Check sheet for the modelled part. Datum: model origin and axes. Units: mm. Face numbers are marked on the shaded views. A direction names the side the tool comes from. Coordinates: 2 decimals unless noted, no trailing zeros. Write each loop counter-clockwise with the first axis right and the second up, starting at its lowest first coordinate (ties: lowest second). Pieces come first, ordered by that corner, then holes. Notation, with made-up numbers: M -29,17.25 L -12,17.25 A27 cw -12,47.25 Z; hole C -1,72.25 d7. An arc over 180 degrees is marked long. Answer as CSV lines item,"result". Start each with the question number.
1) Access from +Z, -Z, +X, -X, +Y, -Y to the whole of each face (thin tool, end or side, straight path). Record for the marked faces 4, 5 and 6.
2) Section check A-A (y = 11). Record the cut outline in (x, z), and give its area (3 significant figures).
3) Draft check along Y on the marked faces 1, 2 and 3. Enter one of: +Y half, -Y half, draft (parallel to the pull), parting line (faces both ways), or undercut.
4) Material ranges on L1, parallel to Z at x = 9, y = 6; L2, parallel to Z at x = 25.5, y = 30.5; L3, parallel to Y at x = 29, z = -9.5, recorded low to high. Write a range as [from, to].
5) Section check C-C (x = 16). Record the cut outline in (y, z).
6) Go/stop test with flat-tipped pins: pin 1 Ø1.4 at (x, z) = (32, -26.5) entering from -Y; pin 2 Ø0.9 at (y, z) = (15.5, -5) entering from +X; pin 3 Ø2 at (x, y) = (15.5, 10.5) entering from -Z. Record where each tip stops, or that it passes through.
7) Section check D-D (y = 31.5). Record the cut outline in (x, z).
8) Section check B-B (z = -20.5). Record the cut outline in (x, y).
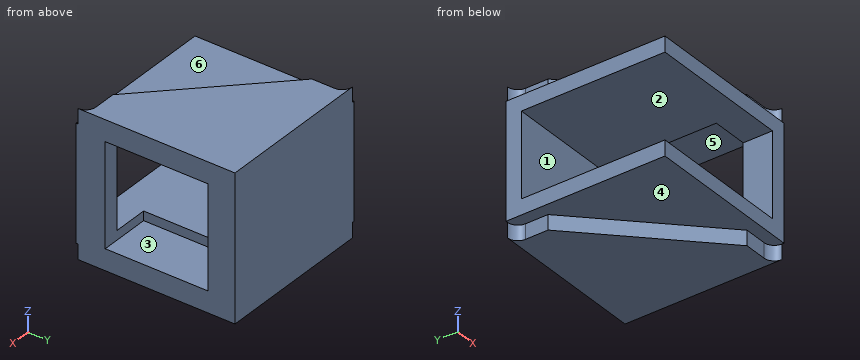
from build123d import *

# Parameters (mm, degrees)
SKETCH_5_W          = 31
SKETCH_5_H          = 31
EXTRUDE_1_DEPTH     = 3
SKETCH_6_W          = 31
SKETCH_6_H          = 31
EXTRUDE_2_DEPTH     = 3
EXTRUDE_3_DEPTH     = 2.9
EXTRUDE_4_DEPTH     = 2.9
EXTRUDE_5_DEPTH     = 16.4
SKETCH_10_W         = 20
SKETCH_10_H         = 20
CUT_EXTRUDE_1_DEPTH = 10


with BuildPart() as part:
    # Sketch 5 → Extrude 1 (new body)
    with BuildSketch(Plane(origin=(835, 815, -2.8), x_dir=(-1, 0, 0), z_dir=(0, 0, 1))):
        with Locations((815.5, 795.5)):
            Rectangle(SKETCH_5_W, SKETCH_5_H)
    extrude(amount=-EXTRUDE_1_DEPTH)

    # Sketch 8 → Extrude 4 (add)
    with BuildSketch(Plane.XY.offset(-2.8)):
        with BuildLine():
            Line((6.4, 33), (6.4, 28.6))
            Line((6.4, 28.6), (28.6, 6.4))
            Line((28.6, 6.4), (33, 6.4))
            ThreePointArc((33, 6.4), (34.414213562, 5.814213562), (35, 4.4))
            Line((35, 4.4), (35, 35))
            Line((35, 35), (4.4, 35))
            ThreePointArc((4.4, 35), (5.814213562, 34.414213562), (6.4, 33))
        make_face()
    extrude(amount=EXTRUDE_4_DEPTH)



with BuildPart() as body_2:
    # Sketch 6 → Extrude 2 (new body)
    with BuildSketch(Plane(origin=(835, 815, -25.2), x_dir=(-1, 0, 0), z_dir=(0, 0, 1))):
        with Locations((815.5, 795.5)):
            Rectangle(SKETCH_6_W, SKETCH_6_H)
    extrude(amount=EXTRUDE_2_DEPTH)

    # Sketch 7 → Extrude 3 (add)
    with BuildSketch(Plane(origin=(0, 0, -25.2), x_dir=(-1, 0, 0), z_dir=(0, 0, -1))):
        with BuildLine():
            Line((-6.4, 28.6), (-28.6, 6.4))
            Line((-28.6, 6.4), (-33, 6.4))
            ThreePointArc((-33, 6.4), (-34.414213562, 5.814213562), (-35, 4.4))
            Line((-35, 4.4), (-35, 35))
            Line((-35, 35), (-4.4, 35))
            ThreePointArc((-4.4, 35), (-5.814213562, 34.414213562), (-6.4, 33))
            Line((-6.4, 33), (-6.4, 28.6))
        make_face()
    extrude(amount=EXTRUDE_3_DEPTH)


with BuildPart() as part_1:
    add(part.part)

    add(body_2.part)  # Extrude 5 merges body 2
    # Sketch 9 → Extrude 5 (add)
    with BuildSketch(Plane(origin=(0, 0, -5.8), x_dir=(-1, 0, 0), z_dir=(0, 0, -1))):
        Polygon((-35, 4), (-32, 4), (-32, 32), (-4, 32), (-4, 35), (-35, 35), align=None)
    extrude(amount=EXTRUDE_5_DEPTH)

    # Sketch 10 → Cut-Extrude 1 (cut)
    with BuildSketch(Plane(origin=(35, 0, 0), x_dir=(0, 0, -1), z_dir=(1, 0, 0))):
        with Locations((14, 19.7)):
            Rectangle(SKETCH_10_W, SKETCH_10_H)
    extrude(amount=-CUT_EXTRUDE_1_DEPTH, mode=Mode.SUBTRACT)


solid = part_1.part
Results found:
1,face 4,"-Z, -X, -Y"
1,face 5,"+X"
1,face 6,"+Z, -X, -Y"
2,outline,"M 4,-25.2 L 24,-25.2 L 24,-28.1 L 35,-28.1 L 35,-24 L 25,-24 L 25,-22.2 L 4,-22.2 Z; M 4,-5.8 L 25,-5.8 L 25,-4 L 35,-4 L 35,0.1 L 24,0.1 L 24,-2.8 L 4,-2.8 Z"
2,area,"214 mm2"
3,face 1,"-Y half"
3,face 2,"draft"
3,face 3,"undercut"
4,L1,"z = [-25.2, -22.2], [-5.8, -2.8]"
4,L2,"z = [-28.1, -22.2], [-5.8, 0.1]"
4,L3,"y = [32, 35]"
5,outline,"M 4,-25.2 L 19,-25.2 L 19,-28.1 L 35,-28.1 L 35,0.1 L 19,0.1 L 19,-2.8 L 4,-2.8 L 4,-5.8 L 32,-5.8 L 32,-22.2 L 4,-22.2 Z"
6,pin 1,"stops at y = 6.4"
6,pin 2,"stops at x = 25"
6,pin 3,"stops at z = -25.2"
7,outline,"M 4,-25.2 L 6.4,-25.2 L 6.4,-28.1 L 35,-28.1 L 35,0.1 L 6.4,0.1 L 6.4,-2.8 L 4,-2.8 L 4,-5.8 L 32,-5.8 L 32,-22.2 L 4,-22.2 Z"
8,outline,"M 4,32 L 32,32 L 32,29.7 L 35,29.7 L 35,35 L 4,35 Z; M 32,4 L 35,4 L 35,9.7 L 32,9.7 Z"
